Model file for the job. Use its own axes, mm. Face numbers are marked on the shaded views. A direction names the side the tool comes from. Coordinates: 2 decimals unless noted, no trailing zeros. Loops run counter-clockwise (first coordinate to the right, second up) from the corner with the lowest first, then second, coordinate; pieces in that order, holes last.
from build123d import *

# Parameters (mm, degrees)
F0_R      = 13.589
F1_DEPTH  = 114.3
F3_DEPTH  = 50.546
F4_R      = 5.0165
F5_DEPTH  = 152.4
F6_R      = 6.731
F7_DEPTH  = 106.934
F8_R      = 5.08
F9_R      = 0.508
F10_W     = 8.001
F10_H     = 42.073292
F11_DEPTH = 17.8308
F12_R     = 12.7
F13_DEPTH = 1.5875


with BuildPart() as f1:
    # F0 (on Right) → F1 (new body)
    with BuildSketch(Plane.YZ):
        Circle(F0_R)
    extrude(amount=-F1_DEPTH)

    # F2 (on Front) → F3 (cut, symmetric)
    with BuildSketch(Plane.XZ):
        Polygon((-11.938, 0.889), (-114.3, 0.889), (-114.3, -0.889), (-11.938, -0.889), (-11.938, 0), align=None)
    extrude(amount=F3_DEPTH, both=True, mode=Mode.SUBTRACT)

    # F4 (on face) → F5 (cut)
    with BuildSketch(Plane.YZ):
        Circle(F4_R)
    extrude(amount=-F5_DEPTH, mode=Mode.SUBTRACT)

    # F6 (on face) → F7 (cut)
    with BuildSketch(Plane(origin=(-11.938, 0, 0), x_dir=(0, -1, 0), z_dir=(-1, 0, 0))):
        Circle(F6_R)
    extrude(amount=F7_DEPTH, mode=Mode.SUBTRACT)

    # F8
    f8_edges = [f1.edges().sort_by_distance(p)[0] for p in [
        (-114.3, 10.115962, 0.889),
        (-114.3, -10.115962, 0.889),
        (-114.3, -10.115962, -0.889),
        (-114.3, 10.115962, -0.889),
    ]]
    fillet(f8_edges, radius=F8_R)

    # F9
    f9_edges = [f1.edges().sort_by_distance(p)[0] for p in [
        (-11.938, 10.115962, 0.889),
        (-11.938, -10.115962, 0.889),
        (-11.938, 10.115962, -0.889),
        (-11.938, -10.115962, -0.889),
        (-11.938, 0, 6.731),
        (-11.938, 0, -6.731),
    ]]
    fillet(f9_edges, radius=F9_R)

    # F10 (on Front) → F11 (cut, symmetric)
    with BuildSketch(Plane.XZ):
        Rectangle(F10_W, F10_H)
    extrude(amount=F11_DEPTH, both=True, mode=Mode.SUBTRACT)

    # F12 (on face) → F13 (cut)
    with BuildSketch(Plane.YZ.offset(-4.0005)):
        Circle(F12_R)
    extrude(amount=-F13_DEPTH, mode=Mode.SUBTRACT)


solid = f1.part
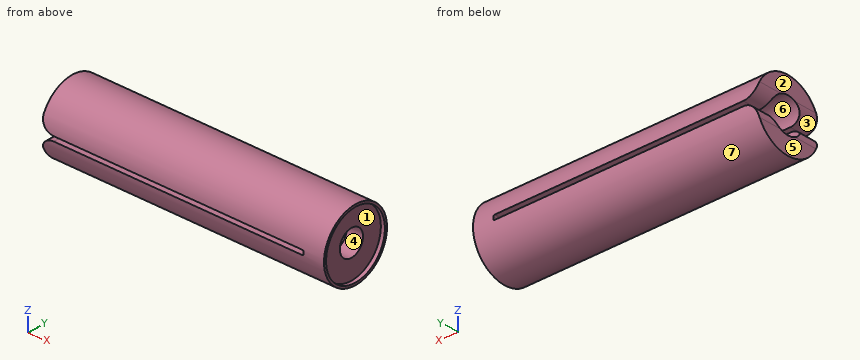
Q1. Drill centre lines: line 1 (Z direction, x = -10.5, y = 0); line 2 (X direction, y = -2, z = -12.25); line 3 (Z direction, x = -14, y = -5.5). Where is each one in solid material? Low to high.
Answers:
line 1: z = -13.59 to -5.02, 5.02 to 13.59
line 2: x = -114.3 to -5.59
line 3: z = -12.43 to -3.88, 3.88 to 12.43
Q2. Slice it at C-C (y = 9.25). List the corners of the cut face in (x, z), and give its area (3 significant figures).
Answers:
outline: (-114.3, -9.95) - (-4, -9.95) - (-4, -8.7) - (-5.59, -8.7) - (-5.59, 8.7) - (-4, 8.7) - (-4, 9.95) - (-114.3, 9.95) - (-114.3, 5.97) arc R5.08 ccw to (-109.22, 0.89) - (-12.45, 0.89) arc R0.51 cw to (-11.94, 0.38) - (-11.94, -0.38) arc R0.51 cw to (-12.45, -0.89) - (-109.22, -0.89) arc R5.08 ccw to (-114.3, -5.97) - close
area: 1,980 mm2
Q3. Flat gauge pins, fed straight in: P1, Ø4, axis at x = -102.5, z = -7.5, coming from the -Y side; P2, Ø4, axis at x = -90.5, z = 6.5, coming from the +Y side; P3, Ø1, axis at y = -7.5, z = 2.5, coming from the -X side. Where does each tip first touch, or does it go through?
Answers:
P1: stops at y = -12.43
P2: stops at y = 12.82
P3: stops at x = -113.34
Q4. Which spindle directions (+Z, -Z, +X, -X, +Y, -Y) get a long thin tool onto all of the face, cutting with end or side? Do the marked faces 1, 2 and 3. Say none if no direction does.
Answers:
face 1: +X
face 2: +Z, -Z, -X, +Y, -Y
face 3: -X, +Y, -Y
Q5. Slice it at B-B (y = 0). List the corners of the cut face in (x, z), and give its area (3 significant figures).
Answers:
outline: (-114.3, -13.59) - (-4, -13.59) - (-4, -12.7) - (-5.59, -12.7) - (-5.59, -5.02) - (-11.94, -5.02) - (-11.94, -6.22) arc R0.51 cw to (-12.45, -6.73) - (-114.3, -6.73) - close; (-114.3, 6.73) - (-12.45, 6.73) arc R0.51 cw to (-11.94, 6.22) - (-11.94, 5.02) - (-5.59, 5.02) - (-5.59, 12.7) - (-4, 12.7) - (-4, 13.59) - (-114.3, 13.59) - close
area: 1,520 mm2
Q6. Mould opens along Z. For the marked faces 4, 5, 6 and 7 say: +Z half, -Z half, draft (parallel to the pull), parting line (faces both ways), or undercut.
Answers:
face 4: undercut
face 5: draft
face 6: undercut
face 7: parting line
Q7. Slice it at A-A (x = -105.5). List the corners of the cut face in (y, z), and give its area (3 significant figures).
Answers:
outline: (-13.56, -0.89) arc R13.59 ccw to (13.56, -0.89) - (6.67, -0.89) arc R6.73 cw to (-6.67, -0.89) - close; (-13.56, 0.89) - (-6.67, 0.89) arc R6.73 cw to (6.67, 0.89) - (13.56, 0.89) arc R13.59 ccw to start
area: 413 mm2
